from build123d import *

# Parameters (mm, degrees)
Y_KSEKLIK_EKSTR_ZYON1_DEPTH = 5
RADYUS1_R                   = 2
IZIM2_R                     = 1.7
KES_EKSTR_ZYON1_DEPTH       = 12
Y_KSEKLIK_EKSTR_ZYON2_DEPTH = 40
PAH1_SIZE                   = 3


with BuildPart() as part:
    # Çizim1 → Yükseklik-Ekstrüzyon1 (new body)
    with BuildSketch(Plane.XY):
        Polygon((0, 0), (10, 0), (10, -50), (5.050252532, -54.949747468), (0, -50), align=None)
    extrude(amount=Y_KSEKLIK_EKSTR_ZYON1_DEPTH)

    # Radyus1
    radyus1_edges = [part.edges().sort_by_distance(p)[0] for p in [
        (0, 0, 2.5),
        (10, 0, 2.5),
    ]]
    fillet(radyus1_edges, radius=RADYUS1_R)

    # Çizim2 → Kes-Ekstrüzyon1 (cut)
    with BuildSketch(Plane.XY.offset(5)):
        with Locations((5, -4)):
            Circle(IZIM2_R)
    extrude(amount=-KES_EKSTR_ZYON1_DEPTH, mode=Mode.SUBTRACT)

    # Çizim3 → Yükseklik-Ekstrüzyon2 (add)
    with BuildSketch(Plane.XZ.offset(50)):
        Polygon((7.5, 10), (2.5, 10), (2.5, -5), (3.3, -5), (7.5, -5), align=None)
    extrude(amount=Y_KSEKLIK_EKSTR_ZYON2_DEPTH)

    # Pah1
    pah1_edges = [part.edges().sort_by_distance(p)[0] for p in [
        (5, -50, 0),
        (5, -50, 5),
    ]]
    chamfer(pah1_edges, length=PAH1_SIZE)


solid = part.part
Can you work these out from the model? Positions are in its coordinate system, mm. A direction names the side the tool comes from. Coordinates: 2 decimals unless noted, no trailing zeros. Loops run counter-clockwise (first coordinate to the right, second up) from the corner with the lowest first, then second, coordinate; pieces in that order, holes last. Notation, with made-up numbers: (2, 71) - (39, 71) arc R18 ccw to (39, 105) - close; hole circle Ø8 at (-9, 25). An arc over 180 degrees is marked (long way). Put each result on its own line as item: value. Start each with the question number.
Item 1: Suppose I cut it at C-C (z = 4). Please give me the cut outline in (x, y), and give its area (3 significant figures).
Item 2: If I drill on line 1 along Y through (x, z) = (5, 1.2); line 2 along Z through (x, y) = (5, -12.5); line 3 along Y through (x, z) = (4.5, 9), over which ranges is the centre line in solid material (lowest first)?
Item 3: Which directions (+Z, -Z, +X, -X, +Y, -Y) give clear straight access to the entire face, cutting with the end or side of a thin tool? Please do faces 1 (the face through (5, 0, 2)), 2 (the face through (5, -50, 9)), 3 (the face through (5, -50, -4)).
Item 4: Suppose I cut it at D-D (z = -2). Please give me the cut outline in (x, y), and give its area (3 significant figures).
Item 5: Suppose I cut it at B-B (x = 5). Please give me the cut outline in (y, z).
Item 6: For pin 1 (3 mm diameter, centred on x = 5, y = -34.5, fed in from +Z); pin 2 (1.6 mm diameter, centred on x = 4.5, z = 9, fed in from +Y); pin 3 (2 mm diameter, centred on x = 6, y = -26.5, fed in from -Z); pin 4 (2.5 mm diameter, centred on x = 5, y = -4, fed in from -Z) (1 decimal), each with a flat end and sliding along its axis, tell me the tip position at first contact or that it passes through.
Item 7: If we mould it in two halves opening along Y, with no side actions, what happens to faces 4 (the face through (9.4, -0.57, 2.54)), 5 (the face through (5.8, -5.5, 2.5)), 6 (the face through (5, -70, 10))? For each: +Y half, -Y half, draft (parallel to the pull), parting line (faces both ways), or undercut.
Item 8: Suppose I cut it at A-A (y = -4). Please give me the cut outline in (x, z).
Here are the results:
1. outline: (0, -50) - (2.5, -52.45) - (2.5, -90) - (7.5, -90) - (7.5, -52.5) - (10, -50) - (10, -2) arc R2 ccw to (8, 0) - (2, 0) arc R2 ccw to (0, -2) - close; hole circle Ø3.4 at (5, -4)
1. area: 695 mm²
2. line 1: -90 to -5.7, -2.3 to 0
2. line 2: 0 to 5
2. line 3: -90 to -50
3. face 1: +Z, -Z, +X, -X, +Y
3. face 2: +Z, +X, -X, +Y
3. face 3: -Z, +X, -X, +Y
4. outline: (2.5, -90) - (7.5, -90) - (7.5, -49) - (2.5, -49) - close
4. area: 205 mm²
5. outline: (-90, -5) - (-50, -5) - (-50, -3) - (-47, 0) - (-5.7, 0) - (-5.7, 5) - (-47, 5) - (-50, 8) - (-50, 10) - (-90, 10) - close; (-2.3, 0) - (0, 0) - (0, 5) - (-2.3, 5) - close
6. pin 1: z = 5
6. pin 2: y = -50
6. pin 3: z = 0
6. pin 4: through
7. face 4: +Y half
7. face 5: undercut
7. face 6: draft
8. outline: (0, 0) - (3.3, 0) - (3.3, 5) - (0, 5) - close; (6.7, 0) - (10, 0) - (10, 5) - (6.7, 5) - close
